Check sheet for the modelled part. Datum: model origin and axes. Units: mm. Face numbers are marked on the shaded views. Coordinates: 2 decimals unless noted, no trailing zeros. Loops run counter-clockwise (first coordinate to the right, second up) from the corner with the lowest first, then second, coordinate; pieces in that order, holes last.
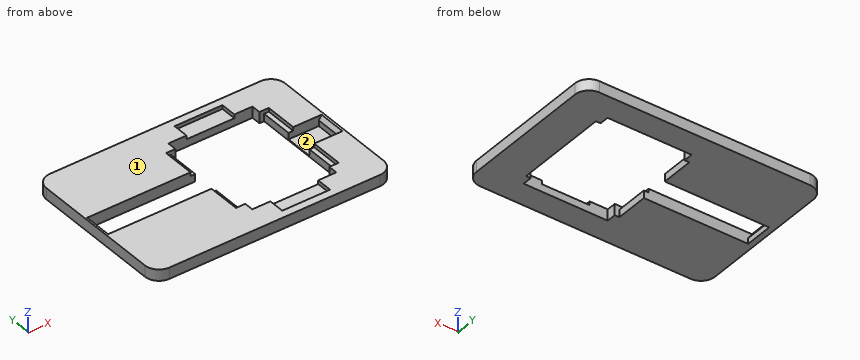
Autodesk Fusion 360 part; units mm, degrees
sketch "Sketch1" plane through (0, 0, 0) normal (0, 0, 1) x (1, 0, 0)
  line L0 (63.855, -42.715) -> (-63.855, -42.715)
  line L1 (-63.855, -42.715) -> (-63.855, 42.715)
  line L2 (-63.855, 42.715) -> (63.855, 42.715)
  line L3 (63.855, 42.715) -> (63.855, -42.715)
  line L4 (63.855, -42.715) -> (-63.855, 42.715) construction
  line L5 (-63.855, -42.715) -> (63.855, 42.715) construction
  line L6 (45, -38.5) -> (-5, -38.5)
  line L7 (-5, -38.5) -> (-5, 38.5)
  line L8 (-5, 38.5) -> (45, 38.5)
  line L9 (45, 38.5) -> (45, -38.5)
  line L10 (45, -38.5) -> (-5, 38.5) construction
  line L11 (-5, -38.5) -> (45, 38.5) construction
  line L12 (-2.5, 30) -> (42.5, 30)
  line L13 (42.5, 30) -> (42.5, -30)
  line L14 (42.5, -30) -> (-2.5, -30)
  line L15 (-2.5, -30) -> (-2.5, 30)
  line L16 (-2.5, 30) -> (42.5, -30) construction
  line L17 (42.5, 30) -> (-2.5, -30) construction
  line L18 (-7.5, 25) -> (47.5, 25)
  line L19 (47.5, 25) -> (47.5, -25)
  line L20 (47.5, -25) -> (-7.5, -25)
  line L21 (-7.5, -25) -> (-7.5, 25)
  line L22 (-7.5, 25) -> (47.5, -25) construction
  line L23 (47.5, 25) -> (-7.5, -25) construction
  line L24 (63.855, 42.715) -> (83.855, 42.715)
  line L25 (83.855, 42.715) -> (83.855, -42.715)
  line L26 (83.855, -42.715) -> (63.855, -42.715)
  line L27 (63.855, -42.715) -> (63.855, 42.715)
  line L28 (-63.855, 42.715) -> (-43.855, 42.715)
  line L29 (-43.855, 42.715) -> (-43.855, -42.715)
  line L30 (-43.855, -42.715) -> (-63.855, -42.715)
  line L31 (-63.855, -42.715) -> (-63.855, 42.715)
  point P0 (20, 0)
  point P1 (20, 0)
  point P2 (20, 0)
  dimension "d1" = 85.43
  dimension "d2" = 127.71
  dimension "d3" = 50
  dimension "d4" = 77
  dimension "d5" = 45
  dimension "d6" = 60
  dimension "d7" = 55
  dimension "d8" = 50
  dimension "d43" = 20
  dimension "d44" = 20
extrude "Extrude1" add sketch "Sketch1" along normal blind 3 contours L0 L2 L3 L27 L29 | L0 L1 L2 L28 L29 L30 L31 makes body 1
extrude "Extrude2" add sketch "Sketch1" along normal blind 1 contours L6 L7 L9 L13 L14 L15 L20 | L9 L18 L19 L20 | L7 L18 L20 L21 | L7 L8 L9 L12 L13 L15 L18 bodies 1
fillet "Fillet1" radius 7.5 4 edges at (-63.855, -42.715, 1.5) (63.855, -42.715, 1.5) (-63.855, 42.715, 1.5) (63.855, 42.715, 1.5) on bodies 1
sketch "Sketch2" plane through (0, 0, 3) normal (0, 0, 1) x (-1, 0, 0)
  line L0 (-56.355, -42.715) -> (56.355, -42.715)
  line L1 (56.355, 42.715) -> (-56.355, 42.715)
  line L2 (5, 25) -> (7.5, 25)
  line L3 (7.5, 25) -> (7.5, -25)
  line L4 (7.5, -25) -> (5, -25)
  line L5 (5, -25) -> (5, -38.5)
  line L6 (5, -38.5) -> (-45, -38.5)
  line L7 (-45, -38.5) -> (-45, -25)
  line L8 (-45, -25) -> (-47.5, -25)
  line L9 (-47.5, -25) -> (-47.5, 25)
  line L10 (-47.5, 25) -> (-45, 25)
  line L11 (-45, 25) -> (-45, 38.5)
  line L12 (-45, 38.5) -> (5, 38.5)
  line L13 (5, 38.5) -> (5, 25)
  line L14 (5, 25) -> (5, 27.5)
  arc A0 (7.5, 25) -> (5, 27.5) centre (3.9613, 23.9613) ccw
  line L15 (-20, 5) -> (-20, 10)
  line L16 (-20, 10) -> (-20, 5)
  line L17 (-20, 5) -> (-15, 5)
  arc A1 (5, -17.5) -> (7.5, -15) centre (3.9613, -13.9613) ccw
  arc A2 (-47.5, -15) -> (-45, -17.5) centre (-43.9613, -13.9613) ccw
  arc A3 (-45, 27.5) -> (-47.5, 25) centre (-43.9613, 23.9613) ccw
  arc A4 (-63.855, -35.215) -> (-56.355, -42.715) centre (-56.355, -35.215) ccw
  arc A5 (56.355, -42.715) -> (63.855, -35.215) centre (56.355, -35.215) ccw
  line L18 (63.855, -35.215) -> (63.855, 35.215)
  arc A6 (63.855, 35.215) -> (56.355, 42.715) centre (56.355, 35.215) ccw
  arc A7 (-56.355, 42.715) -> (-63.855, 35.215) centre (-56.355, 35.215) ccw
  line L19 (-63.855, 35.215) -> (-63.855, -35.215)
  dimension "d14" = 2.5
extrude "Extrude3" [suppressed]
fillet "Fillet2" [suppressed]
ref_plane "WorkPlane1" through (12.125, 0, 0) normal (0, -1, 0) x (1, 0, 0)
sketch "Sketch5" plane through (12.125, 0, 0) normal (0, -1, 0) x (1, 0, 0)
  line L0 (-15, 3) -> (-72.9634, 3)
  line L1 (-72.9634, 3) -> (-72.9634, 0)
  line L2 (-72.9634, 0) -> (-15, 0)
  line L3 (-15, 0) -> (-15, 3)
  line L4 (-72.9634, 0) -> (-74.9634, 3)
  line L5 (-74.9634, 3) -> (-72.9634, 3)
  line L6 (32, 3) -> (49.0623, 3)
  line L7 (49.0623, 3) -> (49.0623, 0.5905)
  line L8 (49.0623, 0.5905) -> (32, 0.5905)
  line L9 (32, 0.5905) -> (32, 3)
  line L10 (49.0623, 0.5905) -> (50.5109, 3)
  line L11 (50.5109, 3) -> (49.0623, 3)
extrude "Extrude5" cut sketch "Sketch5" along normal mid plane 15 bodies 1
extrude "Extrude9" add 1 faces at (-40.7311, -25.0717, 0) along direction (0, 0, -1) blind 3 on bodies 1 bodies 1
extrude "Extrude10" cut 1 faces at (55.7915, 2.5, 0.5905) along direction (0, 0, -1) blind 3 on bodies 1 bodies 1
sketch "Sketch6" plane through (0, 0, 1) normal (0, 0, 1) x (-1, 0, 0)
  line L0 (-45, -25) -> (-45, -38.5)
  line L1 (-45, -38.5) -> (5, -38.5)
  line L2 (5, -38.5) -> (5, -25)
  line L3 (2.5, -25) -> (2.5, -30)
  line L4 (2.5, -30) -> (-42.5, -30)
  line L5 (-42.5, -30) -> (-42.5, -25)
  line L6 (-20, -38.5) -> (-7.2, -38.5)
  line L7 (-20, -38.5) -> (-32.8, -38.5)
  line L8 (-7.2, -38.5) -> (-32.8, -38.5)
  line L9 (-32.8, -38.5) -> (-32.8, 39.8185)
  line L10 (-32.8, 39.8185) -> (-7.2, 39.8185)
  line L11 (-7.2, 39.8185) -> (-7.2, -38.5)
  line L12 (-42.5, -25) -> (-45, -25)
  line L13 (5, -25) -> (2.5, -25)
  dimension "d35" = 12.8
  dimension "d36" = 12.8
extrude "Extrude12" add sketch "Sketch6" along normal blind 2 separate body contours L0 L1 L4 L5 L9 L12 | L1 L2 L3 L4 L11 L13 makes body 2 at (-0.1, 35.6667, 1) makes body 3 at (40.1, 35.6667, 1)
mirror "Mirror1" about plane through (0, 0, 0) normal (0, 1, 0) of bodies 3 2 makes body 4 at (40.1, -35.6667, 1) makes body 5 at (-0.1, -35.6667, 1)
combine "Combine1" operation add target body 5 tool bodies 3 4 1 2
(1) Scan lines: line 1 along X through (y, z) = (-16.5, 1.6) (3 decimals); line 2 along Y through (x, z) = (-51, -0.8) (3 decimals); line 3 along X through (y, z) = (21.5, -1.6) (3 decimals). Record each from-to range of solid material in increasing order.
(2) Gauge pin test, flat ends, axial feed: P1, Ø1.6, axis at x = 58, z = 1.5, coming from the -Y side; P2, Ø1.2, axis at x = -5.5, y = 16.5, coming from the +Z side; P3, Ø10, axis at x = -47.5, y = -3.5, coming from the -Z side. Record the tip position at first contact, or that the pin passes through.
(3) Draft check along Y on the marked faces 1 and 2. Enter one of: pulls with the +Y half, pulls with the -Y half, needs draft (parallel to the pull), parting line crosses it, or undercut.
(4) Section check C-C, the plane x = 28.5. Enter the section's corners in (y, z) (3 decimals).
(5) Section check B-B, the plane y = -17. Enter the section's corners in (x, z) (3 decimals), plus the area to 3 significant figures.
(6) Section check A-A, the plane x = -16. Enter the section's corners in (y, z) (3 decimals).
Determined:
1. line 1: x = -63.855 to -7.5, 47.5 to 63.855
1. line 2: y = -42.715 to -7.5, 7.5 to 42.715
1. line 3: x = -63.855 to -5, 45 to 63.855
2. P1: stops at y = -42.67
2. P2: stops at z = 1
2. P3: stops at z = -3
3. face 1: needs draft
3. face 2: undercut
4. outline: (-42.715, -3) - (-30, -3) - (-30, 1) - (-38.5, 1) - (-38.5, 3) - (-42.715, 3) - close; (30, -3) - (42.715, -3) - (42.715, 3) - (38.5, 3) - (38.5, 1) - (30, 1) - close
5. outline: (-63.855, -3) - (-5, -3) - (-5, 1) - (-7.5, 1) - (-7.5, 3) - (-63.855, 3) - close; (45, -3) - (63.855, -3) - (63.855, 3) - (47.5, 3) - (47.5, 1) - (45, 1) - close
5. area: 456 mm2
6. outline: (-42.715, -3) - (-7.5, -3) - (-7.5, 3) - (-42.715, 3) - close; (7.5, -3) - (42.715, -3) - (42.715, 3) - (7.5, 3) - close
